```python
from build123d import *

# Parameters (mm, degrees)
SKETCH1_R           = 42.5
SKETCH1_R_2         = 24
BOSS_EXTRUDE1_DEPTH = 2
SKETCH3_R           = 3.25
SKETCH3_R_2         = 3.2
CUT_EXTRUDE1_DEPTH  = 2


with BuildPart() as part:
    # Sketch1 → Boss-Extrude1 (new body)
    with BuildSketch(Plane(origin=(0, 0, 0), x_dir=(1, 0, 0), z_dir=(0, 1, 0))):
        with Locations(Location((0, 0, 0), (0, 0, 270))):
            Circle(SKETCH1_R)
        with Locations(Location((0, 0, 0), (0, 0, 270))):
            Circle(SKETCH1_R_2, mode=Mode.SUBTRACT)
    extrude(amount=BOSS_EXTRUDE1_DEPTH)

    # Sketch3 → Cut-Extrude1 (cut)
    with BuildSketch(Plane(origin=(0, 2, 0), x_dir=(1, 0, 0), z_dir=(0, 1, 0))):
        with Locations(Location((0, -31.75, 0), (0, 0, 270))):
            Circle(SKETCH3_R)
        with Locations(Location((-27.49630657, 15.875, 0), (0, 0, 270))):
            Circle(SKETCH3_R)
        with Locations(Location((27.49630657, 15.875, 0), (0, 0, 270))):
            Circle(SKETCH3_R)
        with Locations(Location((0, 34, 0), (0, 0, 270))):
            Circle(SKETCH3_R_2)
        with Locations(Location((29.444863729, -17, 0), (0, 0, 270))):
            Circle(SKETCH3_R_2)
        with Locations(Location((-29.444863729, -17, 0), (0, 0, 270))):
            Circle(SKETCH3_R_2)
    extrude(amount=-CUT_EXTRUDE1_DEPTH, mode=Mode.SUBTRACT)


solid = part.part
```
The listing builds one solid part. Answer for the finished solid, in the listing's coordinates (mm). Coordinates: 2 decimals unless noted, no trailing zeros. Write each loop counter-clockwise with the first axis right and the second up, starting at its lowest first coordinate (ties: lowest second). Pieces come first, ordered by that corner, then holes. Notation, with made-up numbers: M 14.5,-39.75 L 56.5,-39.75 A7 ccw 56.5,-29.75 Z; hole C 38,63 d11. An arc over 180 degrees is marked long. Use a Markdown table: item, result. Add a question column.
1. Section B-B (x = -18) is taken. Give the vertices of the cut face in (y, z).
2. Section A-A (z = -34) is taken. Give the vertices of the cut face in (x, y).
3. Straight lines are drawn through the part: line 1 along X through (y, z) = (1.6, -1); line 2 along Z through (x, y) = (1, 1.05); line 3 along X through (y, z) = (0.85, 17). For each, find the intervals that lie inside material, in ascending order. Write a range as [from, to].
4. For a pull along X with two mould halves and no side action, classify faces 1 (the cylindrical face through (30.72, 1.01, -16.3)), 2 (the cylindrical face through (-27.282, 1.014, 14.641)), 3 (the cylindrical face through (-25.861, 0.986, -33.727)), 4 (the flat face through (-18, 2, 18)) as +X half, -X half, draft (parallel to the pull), parting line (faces both ways), or undercut.
5. Section D-D (z = 17) is taken. Give the vertices of the cut face in (x, y).
6. Given P1, Ø1, axis at x = 22, y = 1, coming from the -Z side, flat-ended and moving along its own axis, determine where the tip first touches the part or whether it passes through.
7. Section C-C (x = 0) is taken. Give the vertices of the cut face in (y, z), plus the area to 3 significant figures.
Data:
| question | item | result |
|---|---|---|
| 1 | outline | M 0,-38.5 L 2,-38.5 L 2,-15.87 L 0,-15.87 Z; M 0,15.87 L 2,15.87 L 2,38.5 L 0,38.5 Z |
| 2 | outline | M -25.5,0 L -3.2,0 L -3.2,2 L -25.5,2 Z; M 3.2,0 L 25.5,0 L 25.5,2 L 3.2,2 Z |
| 3 | line 1 | x = [-42.49, -23.98], [23.98, 42.49] |
| 3 | line 2 | z = [-42.49, -37.04], [-30.96, -23.98], [23.98, 28.66], [34.84, 42.49] |
| 3 | line 3 | x = [-38.95, -32.64], [-26.24, -16.94], [16.94, 26.24], [32.64, 38.95] |
| 4 | face 1 | undercut |
| 4 | face 2 | undercut |
| 4 | face 3 | parting line |
| 4 | face 4 | draft |
| 5 | outline | M -38.95,0 L -32.64,0 L -32.64,2 L -38.95,2 Z; M -26.24,0 L -16.94,0 L -16.94,2 L -26.24,2 Z; M 16.94,0 L 26.24,0 L 26.24,2 L 16.94,2 Z; M 32.64,0 L 38.95,0 L 38.95,2 L 32.64,2 Z |
| 6 | P1 | stops at z = -36.66 |
| 7 | outline | M 0,-42.5 L 2,-42.5 L 2,-37.2 L 0,-37.2 Z; M 0,-30.8 L 2,-30.8 L 2,-24 L 0,-24 Z; M 0,24 L 2,24 L 2,28.5 L 0,28.5 Z; M 0,35 L 2,35 L 2,42.5 L 0,42.5 Z |
| 7 | area | 48.2 mm2 |
